Part model, mm, in its own coordinate system. A direction names the side the tool comes from. Round coordinates to 2 decimals unless told otherwise and drop trailing zeros. Write each loop counter-clockwise with the first axis right and the second up, starting at its lowest first coordinate (ties: lowest second). Pieces come first, ordered by that corner, then holes. Notation, with made-up numbers: (62.5, 15.25) -> (94.5, 15.25) arc R22 cw to (94.5, 28.25) -> close; hole circle Ø3 at (50, 12). An arc over 180 degrees is marked (long way). Return JSON: item names as keys, results as strings. Group by question number.
(1) Drill centre lines: L1, parallel to Z at x = 4.5, y = 0 (3 decimals); L2, parallel to Z at x = 21.7, y = 0 (3 decimals); L3, parallel to Y at x = 17.25, z = 12. Where is each one in solid material? Low to high. Write a range as from..to.
(2) Mould opens along Z. For faces 5 (the flat face through (12.7, -69, -1)), 6 (the cylindrical face through (21.89, -13.77, -61.99)), 7 (the cylindrical face through (6.261, 45.725, -56.141)), 8 (the cylindrical face through (6.26, -64.41, -19.52)) say: +Z half, -Z half, draft (parallel to the pull), parting line (faces both ways), or undercut.
(3) Saw through at B-B (x = 11). List the corners of the cut face in (y, z) (3 decimals), plus the area to 3 significant figures.
(4) Tool access for faces 1 (the flat face through (12.7, 36, -59)), 2 (the flat face through (20.32, 56, -23)), 3 (the flat face through (12.7, 33, 61)), 4 (the cylindrical face through (6.26, 25.9, -67.73)): list every direction of +Z, -Z, +X, -X, +Y, -Y with a clear straight run to the whole face (end or side of a thin tool).
(5) Saw through at A-A (y = 0). List the corners of the cut face in (x, z) (3 decimals), plus the area to 3 significant figures.
(6) Drop flat-ended pins along their axis: pin 1 Ø10 at (y, z) = (-73.5, -11.5) entering from +X; pin 2 Ø12 at (x, y) = (16, 12.5) entering from +Z; pin 3 Ø5 at (x, z) = (10.5, -21) entering from +Y. Give the stop position or say it passes through.
(7) Saw through at C-C (y = -72.39). List the corners of the cut face in (x, z), plus the area to 3 significant figures.
from build123d import *

# Parameters (mm, degrees)
BOSS_EXTRUDE1_DEPTH     = 12.7
F_1_4_CLEARANCE_HOLE1_D = 6.5278
CIRPATTERN1_COUNT       = 3
CHAMFER1_SIZE2          = 1.744648161
CHAMFER1_SIZE           = 0.635


with BuildPart() as part:
    # Sketch1 → Revolve1 (revolve)
    with BuildSketch(Plane.XY):
        Polygon((0, 66.675), (23.495, 66.675), (23.495, 63.5), (20.32, 63.5), (20.32, 60.325), (0, 60.325), align=None)
    revolve(axis=Axis((0, 0, 0), (1, 0, 0)))

    # Sketch5 → Boss-Extrude1 (add)
    with BuildSketch(Plane.ZY):
        with BuildLine():
            ThreePointArc((-61.733643772, 45.671707505), (-70.940470951, 40.9575), (-70.41968082, 30.627050022))
            ThreePointArc((-70.41968082, 30.627050022), (-67.700076965, 25.827577718), (-66.080812198, 20.554138506))
            ThreePointArc((-66.080812198, 20.554138506), (-65.542300069, 15.371802621), (-65.894280688, 10.17346537))
            ThreePointArc((-65.894280688, 10.17346537), (-57.742243797, 33.3375), (-41.757619799, 51.979388355))
            ThreePointArc((-41.757619799, 51.979388355), (-46.083521606, 49.075395572), (-50.840812198, 46.950592813))
            ThreePointArc((-50.840812198, 46.950592813), (-56.217376905, 45.716197631), (-61.733643772, 45.671707505))
        make_face()
    boss_extrude1 = extrude(amount=-BOSS_EXTRUDE1_DEPTH)

    # 1/4 Clearance Hole1 (through all)
    with Locations(Plane.ZY):
        with Locations((-62.69157898, 36.195)):
            f_1_4_clearance_hole1 = Hole(F_1_4_CLEARANCE_HOLE1_D / 2)

    # CirPattern1: Boss-Extrude1, 1/4 Clearance Hole1 ×3 about axis
    cirpattern1_axis = Axis((0, 0, 0), (1, 0, 0))
    for i in range(1, CIRPATTERN1_COUNT):
        add(boss_extrude1.rotate(cirpattern1_axis, i * 360 / CIRPATTERN1_COUNT))
        add(f_1_4_clearance_hole1.rotate(cirpattern1_axis, i * 360 / CIRPATTERN1_COUNT), mode=Mode.SUBTRACT)

    # Chamfer1
    chamfer1_edges = [part.edges().sort_by_distance(p)[0] for p in [
        (0, -60.325, 0),
    ]]
    chamfer(chamfer1_edges, length=CHAMFER1_SIZE, length2=CHAMFER1_SIZE2)


solid = part.part
Computed values:
{
 "1": {"L1": "-66.675..-60.325, 60.325..66.675", "L2": "-66.675..-63.5, 63.5..66.675", "L3": "-65.59..-59.12, 59.12..65.59"},
 "2": {"face 5": "draft", "face 6": "undercut", "face 7": "undercut", "face 8": "-Z half"},
 "3": {"outline": "(-76.299, -8.686) arc R25.4 cw to (-67.505, -15.24) arc R30.48 cw to (-62.153, -24.137) arc R66.675 ccw to (10.173, -65.894) arc R30.48 cw to (20.554, -66.081) arc R25.4 cw to (30.627, -70.42) arc R9.525 ccw to (45.672, -61.734) arc R25.4 cw to (46.951, -50.841) arc R30.48 cw to (51.979, -41.758) arc R66.675 ccw to (51.979, 41.758) arc R30.48 cw to (46.951, 50.841) arc R25.4 cw to (45.672, 61.734) arc R9.525 ccw to (30.627, 70.42) arc R25.4 cw to (20.554, 66.081) arc R30.48 cw to (10.173, 65.894) arc R66.675 ccw to (-62.153, 24.137) arc R30.48 cw to (-67.505, 15.24) arc R25.4 cw to (-76.299, 8.686) arc R9.525 ccw to start; hole circle Ø6.528 at (-72.39, 0); hole circle Ø120.65 at (0, 0); hole circle Ø6.528 at (36.195, -62.692); hole circle Ø6.528 at (36.195, 62.692)", "area": "3,420 mm2"},
 "4": {"face 1": "-Z, +X, +Y", "face 2": "+X", "face 3": "+Z, +X, +Y", "face 4": "-Z, +X, -X"},
 "5": {"outline": "(0, -66.675) -> (23.495, -66.675) -> (23.495, -63.5) -> (20.32, -63.5) -> (20.32, -60.325) -> (1.745, -60.325) -> (0, -60.96) -> close; (0, 60.96) -> (1.745, 60.325) -> (20.32, 60.325) -> (20.32, 63.5) -> (23.495, 63.5) -> (23.495, 66.675) -> (0, 66.675) -> close", "area": "277 mm2"},
 "6": {"pin 1": "x = 12.7", "pin 2": "z = 66.36", "pin 3": "y = 64.06"},
 "7": {"outline": "(0, -10.88) -> (12.7, -10.88) -> (12.7, -3.26) -> (0, -3.26) -> close; (0, 3.26) -> (12.7, 3.26) -> (12.7, 10.88) -> (0, 10.88) -> close", "area": "193 mm2"}
}
